```python
from build123d import *

# Parameters (mm, degrees)
SKETCH2_W           = 470
SKETCH2_H           = 300
BOSS_EXTRUDE1_DEPTH = 5
SKETCH3_R           = 4.05
CUT_EXTRUDE1_DEPTH  = 10
SKETCH4_R           = 9
SKETCH4_R_2         = 2.1
CUT_EXTRUDE2_DEPTH  = 11
SKETCH5_R           = 4.05
CUT_EXTRUDE3_DEPTH  = 11
SKETCH7_R           = 19.1
CUT_EXTRUDE5_DEPTH  = 3
SKETCH8_R           = 15
CUT_EXTRUDE6_DEPTH  = 8
SKETCH9_R           = 2.1
CUT_EXTRUDE7_DEPTH  = 11


with BuildPart() as part:
    # Sketch2 → Boss-Extrude1 (new body, symmetric)
    with BuildSketch(Plane.XY):
        Rectangle(SKETCH2_W, SKETCH2_H)
    extrude(amount=BOSS_EXTRUDE1_DEPTH, both=True)

    # Sketch3 → Cut-Extrude1 (cut)
    with BuildSketch(Plane.XY.offset(5)):
        with Locations((-215, -75)):
            Circle(SKETCH3_R)
        with Locations((-215, -135)):
            Circle(SKETCH3_R)
        with Locations((215, -75)):
            Circle(SKETCH3_R)
        with Locations((215, -135)):
            Circle(SKETCH3_R)
        with Locations((-215, 135)):
            Circle(SKETCH3_R)
        with Locations((215, 135)):
            Circle(SKETCH3_R)
    extrude(amount=-CUT_EXTRUDE1_DEPTH, mode=Mode.SUBTRACT)

    # Sketch4 → Cut-Extrude2 (cut, through all)
    with BuildSketch(Plane.XY.offset(5)):
        with Locations((112.65, 129.5)):
            Circle(SKETCH4_R)
        with Locations((112.65, 35)):
            Circle(SKETCH4_R)
        with Locations((92.65, 129.5)):
            Circle(SKETCH4_R_2)
        with Locations((132.65, 129.5)):
            Circle(SKETCH4_R_2)
        with Locations((132.65, 35)):
            Circle(SKETCH4_R_2)
        with Locations((92.65, 35)):
            Circle(SKETCH4_R_2)
    extrude(amount=-CUT_EXTRUDE2_DEPTH, mode=Mode.SUBTRACT)

    # Sketch5 → Cut-Extrude3 (cut, through all)
    with BuildSketch(Plane.XY.offset(5)):
        with Locations((152.65, 135)):
            Circle(SKETCH5_R)
        with Locations((152.65, 35)):
            Circle(SKETCH5_R)
    extrude(amount=-CUT_EXTRUDE3_DEPTH, mode=Mode.SUBTRACT)

    # Sketch7 → Cut-Extrude5 (cut)
    with BuildSketch(Plane.XY.offset(5)):
        with Locations((112.05, 82.25)):
            Circle(SKETCH7_R)
    extrude(amount=-CUT_EXTRUDE5_DEPTH, mode=Mode.SUBTRACT)

    # Sketch8 → Cut-Extrude6 (cut, through all)
    with BuildSketch(Plane.XY.offset(2)):
        with Locations((112.05, 82.25)):
            Circle(SKETCH8_R)
    extrude(amount=-CUT_EXTRUDE6_DEPTH, mode=Mode.SUBTRACT)

    # Sketch9 → Cut-Extrude7 (cut, through all)
    with BuildSketch(Plane.XY.offset(5)):
        with Locations((88.45, 105.85)):
            Circle(SKETCH9_R)
        with Locations((135.65, 105.85)):
            Circle(SKETCH9_R)
        with Locations((135.65, 58.65)):
            Circle(SKETCH9_R)
        with Locations((88.45, 58.65)):
            Circle(SKETCH9_R)
    extrude(amount=-CUT_EXTRUDE7_DEPTH, mode=Mode.SUBTRACT)


solid = part.part
```
Check sheet for the modelled part. Datum: model origin and axes. Units: mm. A direction names the side the tool comes from. Round coordinates to 2 decimals unless told otherwise and drop trailing zeros. Loops run counter-clockwise (first coordinate to the right, second up) from the corner with the lowest first, then second, coordinate; pieces in that order, holes last. Notation, with made-up numbers: (85.25, 1) - (104.25, 1) arc R10 ccw to (104.25, 18) - close; hole circle Ø10 at (70, 46). An arc over 180 degrees is marked (long way). Write item = value, one per line. Start each with the question number.
Q1. Release check for a two-part mould opening along Y. For faces 1 (the face through (-3, 150, 0)), 2 (the face through (107.909, 63.604, 3.521)), 3 (the face through (235, -2, 0)) record: pulls with the +Y half, pulls with the -Y half, needs draft (parallel to the pull), parting line crosses it, or undercut.
Q2. Thickness scan on L1, parallel to Y at x = 92.65, z = -2.5; L2, parallel to Y at x = 112.65, z = -1; L3, parallel to Y at x = 215, z = -0.5. Record the ranges inside material, lowest first.
Q3. Access from +Z, -Z, +X, -X, +Y, -Y to the whole of each face (thin tool, end or side, straight path). Record for faces 4 (the face through (120.4, 69.6, 2)), 5 (the face through (100.15, 73.12, -1.45)).
Q4. Section check A-A (y = 82.25). Record the boundary of the cut face in (x, z).
Derived:
q1.face_1 = pulls with the +Y half
q1.face_2 = undercut
q1.face_3 = needs draft
q2.L1 = -150 to 32.9, 37.1 to 127.4, 131.6 to 150
q2.L2 = -150 to 26, 44 to 67.26, 97.24 to 120.5, 138.5 to 150
q2.L3 = -150 to -139.05, -130.95 to -79.05, -70.95 to 130.95, 139.05 to 150
q3.face_4 = +Z
q3.face_5 = +Z, -Z
q4.outline = (-235, -5) - (97.05, -5) - (97.05, 2) - (92.95, 2) - (92.95, 5) - (-235, 5) - close; (127.05, -5) - (235, -5) - (235, 5) - (131.15, 5) - (131.15, 2) - (127.05, 2) - close
